Build history of the part. All positions in model axes, mm. A direction names the side the tool comes from. Coordinates: 2 decimals unless noted, no trailing zeros. Loops run counter-clockwise (first coordinate to the right, second up) from the corner with the lowest first, then second, coordinate; pieces in that order, holes last.
(1) Slice it at B-B (z = 9). Give the number of separate pieces and of enclosed holes in the cut face, and give its area (3 significant figures).
(2) Wall check: L1, parallel to X at y = -34, z = 11; L2, parallel to Y at x = 0, z = 16; L3, parallel to X at y = -47, z = 11. Give the ranges that are in metal, low to high.
(3) Tool access for faces 4 (the face through (-41, -50, 11)), 5 (the face through (28.99, 14.85, 22.18)), 6 (the face through (0, -7.681, 34)): list every direction of +Z, -Z, +X, -X, +Y, -Y with a clear straight run to the whole face (end or side of a thin tool).
(4) Slice it at A-A (x = 3.5). Give the cut face in (y, z).
(5) Slice it at C-C (z = 38). Give the cut face in (x, y).
(6) Flat gauge pins, fed straight in: P1, Ø1.5, axis at y = -13, z = 22.5, coming from the -X side; P2, Ø1.5, axis at x = -5.5, z = 22.5, coming from the +Y side; P3, Ø3, axis at y = -15, z = 15, coming from the -X side. Where does each tip first touch, or does it go through?
(7) Slice it at D-D (y = 3.5). Give the cut face in (x, z).
(8) Two-plate mould, pull along Z, no slides. Class faces 1 (the face through (-37.625, -35.788, 7.223)), 2 (the face through (-29.291, -50.515, 11.092)), 3 (the face through (-43.698, -34.19, 21.598)): pulls with the +Z half, pulls with the -Z half, needs draft (parallel to the pull), parting line crosses it, or undercut.
from build123d import *

# Parameters (mm, degrees)
F1_DEPTH      = 45
F2_R          = 4.125
F3_DEPTH      = 10
F4_R          = 4.125
F5_DEPTH      = 10
F6_R          = 4.125
F7_DEPTH      = 20
F9_DEPTH      = 3
F10_R         = 18
F11_W         = 72.4435358676
F11_H         = 36.0539390085
F12_DEPTH     = 100
F13_T1_DEPTH  = 22.5
F13_T6_DEPTH  = 22.5
F13_T12_DEPTH = 22.5
F13_T18_DEPTH = 22.5
F13_T25_DEPTH = 22.5
F13_T31_DEPTH = 22.5
F13_T34_DEPTH = 23.5
F13_T36_DEPTH = 23.5
F13_T38_DEPTH = 25
F13_T40_DEPTH = 25
F14_R         = 10


# Not quite as in the source:
# - a fillet or chamfer that OpenCascade refuses, or shapes differently, is made with other operations: its cross-section is extruded or revolved along the edge and cut away or added


with BuildPart() as f1:
    # F0 (on Top) → F1 (new body)
    with BuildSketch(Plane.XY):
        with BuildLine():
            Line((29.6984848098, 29.6984848098), (0, 0))
            Line((0, 0), (-29.6984848098, 29.6984848098))
            Line((-29.6984848098, 29.6984848098), (-36.7695526217, 22.627416998))
            Line((-36.7695526217, 22.627416998), (-4.4122546938, -9.7298809299))
            ThreePointArc((-4.4122546938, -9.7298809299), (-19.5013094439, -16.4320762481), (-28.9093081896, -30))
            ThreePointArc((-28.9093081896, -30), (-30.0334813831, -34.1915496034), (-30.5532011416, -38.5))
            Line((-30.5532011416, -38.5), (-21.53782951, -38.5))
            ThreePointArc((-21.53782951, -38.5), (21.59, -40), (-21.53782951, -41.5))
            Line((-21.53782951, -41.5), (-30.5532011416, -41.5))
            ThreePointArc((-30.5532011416, -41.5), (-30.0334813831, -45.8084503966), (-28.9093081896, -50))
            ThreePointArc((-28.9093081896, -50), (23.5679237519, -59.5013094439), (4.4122546938, -9.7298809299))
            Line((4.4122546938, -9.7298809299), (36.7695526217, 22.627416998))
            Line((36.7695526217, 22.627416998), (29.6984848098, 29.6984848098))
        make_face()
        with BuildLine():
            ThreePointArc((-30.5532011416, -38.5), (-30.0334813831, -34.1915496034), (-28.9093081896, -30))
            Line((-28.9093081896, -30), (-44.5532011416, -30))
            Line((-44.5532011416, -30), (-44.5532011416, -38.5))
            Line((-44.5532011416, -38.5), (-30.5532011416, -38.5))
        make_face()
        with BuildLine():
            Line((-44.5532011416, -50), (-28.9093081896, -50))
            ThreePointArc((-28.9093081896, -50), (-30.0334813831, -45.8084503966), (-30.5532011416, -41.5))
            Line((-30.5532011416, -41.5), (-44.5532011416, -41.5))
            Line((-44.5532011416, -41.5), (-44.5532011416, -50))
        make_face()
    extrude(amount=F1_DEPTH)

    # F2 (on face) → F3 (cut, through all)
    with BuildSketch(Plane(origin=(0, 0, 0), x_dir=(-0.7071067812, -0.7071067812, 0), z_dir=(-0.7071067812, 0.7071067812, 0))):
        with Locations((-25.4, 15)):
            Circle(F2_R)
    extrude(amount=-F3_DEPTH, mode=Mode.SUBTRACT)

    # F4 (on face) → F5 (cut, through all)
    with BuildSketch(Plane(origin=(0, 0, 0), x_dir=(-0.7071067812, 0.7071067812, 0), z_dir=(0.7071067812, 0.7071067812, 0))):
        with Locations((25.4, 15)):
            Circle(F4_R)
    extrude(amount=-F5_DEPTH, mode=Mode.SUBTRACT)

    # F6 (on face) → F7 (cut, through all)
    with BuildSketch(Plane.XZ.offset(50)):
        with Locations((-36.7312546656, 33.75)):
            Circle(F6_R)
        with Locations((-36.7312546656, 11.25)):
            Circle(F6_R)
    extrude(amount=-F7_DEPTH, mode=Mode.SUBTRACT)

    # F8 (on face) → F9 (cut)
    with BuildSketch(Plane(origin=(0, -30, 0), x_dir=(-1, 0, 0), z_dir=(0, 1, 0))):
        Polygon((43.6562546656, 37.7481506141), (36.7312546656, 41.7463012283), (29.8062546656, 37.7481506141), (29.8062546656, 29.7518493859), (36.7312546656, 25.7536987717), (43.6562546656, 29.7518493859), align=None)
        Polygon((43.6562546656, 7.2518493859), (43.6562546656, 15.2481506141), (36.7312546656, 19.2463012283), (29.8062546656, 15.2481506141), (29.8062546656, 7.2518493859), (36.7312546656, 3.2536987717), align=None)
    extrude(amount=-F9_DEPTH, mode=Mode.SUBTRACT)

    # F10
    f10_edges = [f1.edges().sort_by_distance(p)[0] for p in [
        (-4.412255, -9.729881, 22.5),
        (4.412255, -9.729881, 22.5),
    ]]
    fillet(f10_edges, radius=F10_R)

    # F11 (on Right) → F12 (cut, symmetric)
    with BuildSketch(Plane.YZ):
        with Locations((-43.9025410381, 40.5269695042)):
            Rectangle(F11_W, F11_H)
    extrude(amount=F12_DEPTH, both=True, mode=Mode.SUBTRACT)

    # F13: fillet of radius 3 on 10 edges, made by hand

    # F13_s2 → F13_t1 (join)
    with BuildSketch(Plane.XY):
        with BuildLine():
            ThreePointArc((-28.206162374, -51.8389401608), (-29.3115301597, -50.5016826145), (-30.9723764022, -50))
            Line((-30.9723764022, -50), (-28.9093081896, -50))
            ThreePointArc((-28.9093081896, -50), (-28.5725334833, -50.9251283904), (-28.206162374, -51.8389401608))
        make_face()
    extrude(amount=F13_T1_DEPTH)


with BuildPart() as f13_tool4:
    # F13_s5 → F13_t6 (new body)
    with BuildSketch(Plane.XY):
        with BuildLine():
            ThreePointArc((-28.206162374, -28.1610598392), (-29.3115301597, -29.4983173855), (-30.9723764022, -30))
            Line((-30.9723764022, -30), (-28.9093081896, -30))
            ThreePointArc((-28.9093081896, -30), (-28.5725334833, -29.0748716096), (-28.206162374, -28.1610598392))
        make_face()
    extrude(amount=F13_T6_DEPTH)

    split(bisect_by=Plane(origin=(-10.5917065627, 0, 18.3453739054), x_dir=(0, 1, 0), z_dir=(0.5, 0, -0.8660254038)), keep=Keep.TOP)

    split(bisect_by=Plane.YZ.offset(-29.8062546656), keep=Keep.TOP)


with BuildPart() as f1_1:
    add(f1.part)

    # F13_t3: union F13_tool4
    add(f13_tool4.part)


with BuildPart() as f13_tool10:
    # F13_s11 → F13_t12 (new body)
    with BuildSketch(Plane.XY):
        with BuildLine():
            ThreePointArc((-28.206162374, -28.1610598392), (-29.3115301597, -29.4983173855), (-30.9723764022, -30))
            Line((-30.9723764022, -30), (-28.9093081896, -30))
            ThreePointArc((-28.9093081896, -30), (-28.5725334833, -29.0748716096), (-28.206162374, -28.1610598392))
        make_face()
    extrude(amount=F13_T12_DEPTH)

    split(bisect_by=Plane(origin=(-10.5917065627, 0, 18.3453739054), x_dir=(0, 1, 0), z_dir=(0.5, 0, -0.8660254038)), keep=Keep.TOP)

    split(bisect_by=Plane.YZ.offset(-29.8062546656), keep=Keep.BOTTOM)


with BuildPart() as f1_2:
    add(f1_1.part)

    # F13_t9: union F13_tool10
    add(f13_tool10.part)


with BuildPart() as f13_tool16:
    # F13_s17 → F13_t18 (new body)
    with BuildSketch(Plane.XY):
        with BuildLine():
            ThreePointArc((-28.206162374, -28.1610598392), (-29.3115301597, -29.4983173855), (-30.9723764022, -30))
            Line((-30.9723764022, -30), (-28.9093081896, -30))
            ThreePointArc((-28.9093081896, -30), (-28.5725334833, -29.0748716096), (-28.206162374, -28.1610598392))
        make_face()
    extrude(amount=F13_T18_DEPTH)

    split(bisect_by=Plane(origin=(-10.5917065627, 0, 18.3453739054), x_dir=(0, 1, 0), z_dir=(-0.5, 0, 0.8660254038)), keep=Keep.TOP)

    split(bisect_by=Plane.YZ.offset(-29.8062546656), keep=Keep.TOP)

    split(bisect_by=Plane(origin=(-0.8489207701, 0, -1.4703739054), x_dir=(0, 1, 0), z_dir=(-0.5, 0, -0.8660254038)), keep=Keep.TOP)


with BuildPart() as f1_3:
    add(f1_2.part)

    # F13_t15: union F13_tool16
    add(f13_tool16.part)


with BuildPart() as f13_tool23:
    # F13_s24 → F13_t25 (new body)
    with BuildSketch(Plane.XY):
        with BuildLine():
            ThreePointArc((-28.206162374, -28.1610598392), (-29.3115301597, -29.4983173855), (-30.9723764022, -30))
            Line((-30.9723764022, -30), (-28.9093081896, -30))
            ThreePointArc((-28.9093081896, -30), (-28.5725334833, -29.0748716096), (-28.206162374, -28.1610598392))
        make_face()
    extrude(amount=F13_T25_DEPTH)

    split(bisect_by=Plane.YZ.offset(-29.8062546656), keep=Keep.TOP)

    split(bisect_by=Plane(origin=(-0.8489207701, 0, -1.4703739054), x_dir=(0, 1, 0), z_dir=(0.5, 0, 0.8660254038)), keep=Keep.TOP)


with BuildPart() as f1_4:
    add(f1_3.part)

    # F13_t22: union F13_tool23
    add(f13_tool23.part)


with BuildPart() as f13_tool29:
    # F13_s30 → F13_t31 (new body)
    with BuildSketch(Plane.XY):
        with BuildLine():
            ThreePointArc((-28.206162374, -28.1610598392), (-29.3115301597, -29.4983173855), (-30.9723764022, -30))
            Line((-30.9723764022, -30), (-28.9093081896, -30))
            ThreePointArc((-28.9093081896, -30), (-28.5725334833, -29.0748716096), (-28.206162374, -28.1610598392))
        make_face()
    extrude(amount=F13_T31_DEPTH)

    split(bisect_by=Plane.YZ.offset(-29.8062546656), keep=Keep.BOTTOM)

    split(bisect_by=Plane(origin=(-0.8489207701, 0, -1.4703739054), x_dir=(0, 1, 0), z_dir=(0.5, 0, 0.8660254038)), keep=Keep.TOP)


with BuildPart() as f1_5:
    add(f1_4.part)

    # F13_t28: union F13_tool29
    add(f13_tool29.part)

    # F13_s35 → F13_t34 (cut)
    with BuildSketch(Plane.XZ.offset(34)):
        with BuildLine():
            ThreePointArc((-44.5532011416, 3), (-43.6745214852, 0.8786796564), (-41.5532011416, 0))
            Line((-41.5532011416, 0), (-44.5532011416, 0))
            Line((-44.5532011416, 0), (-44.5532011416, 3))
        make_face()
        with BuildLine():
            ThreePointArc((-44.5532011416, 19.5), (-43.6745214852, 21.6213203436), (-41.5532011416, 22.5))
            Line((-41.5532011416, 22.5), (-44.5532011416, 22.5))
            Line((-44.5532011416, 22.5), (-44.5532011416, 19.5))
        make_face()
    extrude(amount=F13_T34_DEPTH, mode=Mode.SUBTRACT)

    # F13_s37 → F13_t36 (cut)
    with BuildSketch(Plane.XZ.offset(22.5)):
        with BuildLine():
            ThreePointArc((-44.5532011416, 3), (-43.6745214852, 0.8786796564), (-41.5532011416, 0))
            Line((-41.5532011416, 0), (-44.5532011416, 0))
            Line((-44.5532011416, 0), (-44.5532011416, 3))
        make_face()
        with BuildLine():
            ThreePointArc((-44.5532011416, 19.5), (-43.6745214852, 21.6213203436), (-41.5532011416, 22.5))
            Line((-41.5532011416, 22.5), (-44.5532011416, 22.5))
            Line((-44.5532011416, 22.5), (-44.5532011416, 19.5))
        make_face()
    extrude(amount=F13_T36_DEPTH, mode=Mode.SUBTRACT)

    # F13_s39 → F13_t38 (cut)
    with BuildSketch(Plane(origin=(5.3033008589, 5.3033008589, 0), x_dir=(0, 0, 1), z_dir=(-0.7071067812, -0.7071067812, 0))):
        with BuildLine():
            ThreePointArc((42, 42), (44.1213203436, 41.1213203436), (45, 39))
            Line((45, 39), (45, 42))
            Line((45, 42), (42, 42))
        make_face()
        with BuildLine():
            ThreePointArc((3, 42), (0.8786796564, 41.1213203436), (0, 39))
            Line((0, 39), (0, 42))
            Line((0, 42), (3, 42))
        make_face()
    extrude(amount=F13_T38_DEPTH, mode=Mode.SUBTRACT)

    # F13_s41 → F13_t40 (cut)
    with BuildSketch(Plane(origin=(12.3743686708, -12.3743686708, 0), x_dir=(0, 0, 1), z_dir=(-0.7071067812, 0.7071067812, 0))):
        with BuildLine():
            ThreePointArc((45, 39), (44.1213203436, 41.1213203436), (42, 42))
            Line((42, 42), (45, 42))
            Line((45, 42), (45, 39))
        make_face()
        with BuildLine():
            ThreePointArc((3, 42), (0.8786796564, 41.1213203436), (0, 39))
            Line((0, 39), (0, 42))
            Line((0, 42), (3, 42))
        make_face()
    extrude(amount=F13_T40_DEPTH, mode=Mode.SUBTRACT)

    # F14
    f14_edges = [f1_5.edges().sort_by_distance(p)[0] for p in [
        (-16.296581, -7.680773, 33.75),
        (16.296581, -7.680773, 33.75),
    ]]
    fillet(f14_edges, radius=F14_R)


solid = f1_5.part
Response values:
1. separate pieces: 3
1. enclosed holes: 0
1. area: 2,690 mm2
2. L1: x = -44.55 to -40.85, -32.61 to -20.74, 20.74 to 30
2. L2: y = -70.59 to -61.59, -18.41 to 0
2. L3: x = -44.55 to -40.85, -32.61 to -20.42, 20.42 to 29.78
3. face 4: +Z, -Z, -X, -Y
3. face 5: +Z, -Z, +X
3. face 6: +Z, +X, -X, -Y
4. outline: (-70.39, 0) - (-61.3, 0) - (-61.3, 22.5) - (-70.39, 22.5) - close; (-18.7, 0) - (3.5, 0) - (3.5, 45) - (-7.68, 45) - (-7.68, 22.5) - (-18.7, 22.5) - close
5. outline: (-36.77, 22.63) - (-21.43, 7.29) arc R18 cw to (-16.86, -0.45) arc R10 ccw to (-7.25, -7.68) - (7.25, -7.68) arc R10 ccw to (16.86, -0.45) arc R18 cw to (21.43, 7.29) - (36.77, 22.63) - (29.7, 29.7) - (0, 0) - (-29.7, 29.7) - close
6. P1: stops at x = -18.19
6. P2: stops at y = 6.25
6. P3: stops at x = -19.95
7. outline: (-18.53, 0) - (-3.5, 0) - (-3.5, 45) - (-18.53, 45) - close; (3.5, 0) - (18.53, 0) - (18.53, 45) - (3.5, 45) - close
8. face 1: undercut
8. face 2: needs draft
8. face 3: pulls with the +Z half
